Geometry check sheet. Reference: drawing and pictorial views, mm from the part's lowest x, y, z. A direction names the side the tool comes from. Round coordinates to 2 decimals unless told otherwise and drop trailing zeros. Write each loop counter-clockwise with the first axis right and the second up, starting at its lowest first coordinate (ties: lowest second). Pieces come first, ordered by that corner, then holes. Notation, with made-up numbers: M 57,-31 L 85,-31 A12 ccw 85,-23 Z; hole C -23.75,-36 d7. An arc over 180 degrees is marked long. Answer in a Markdown table with one row per item.
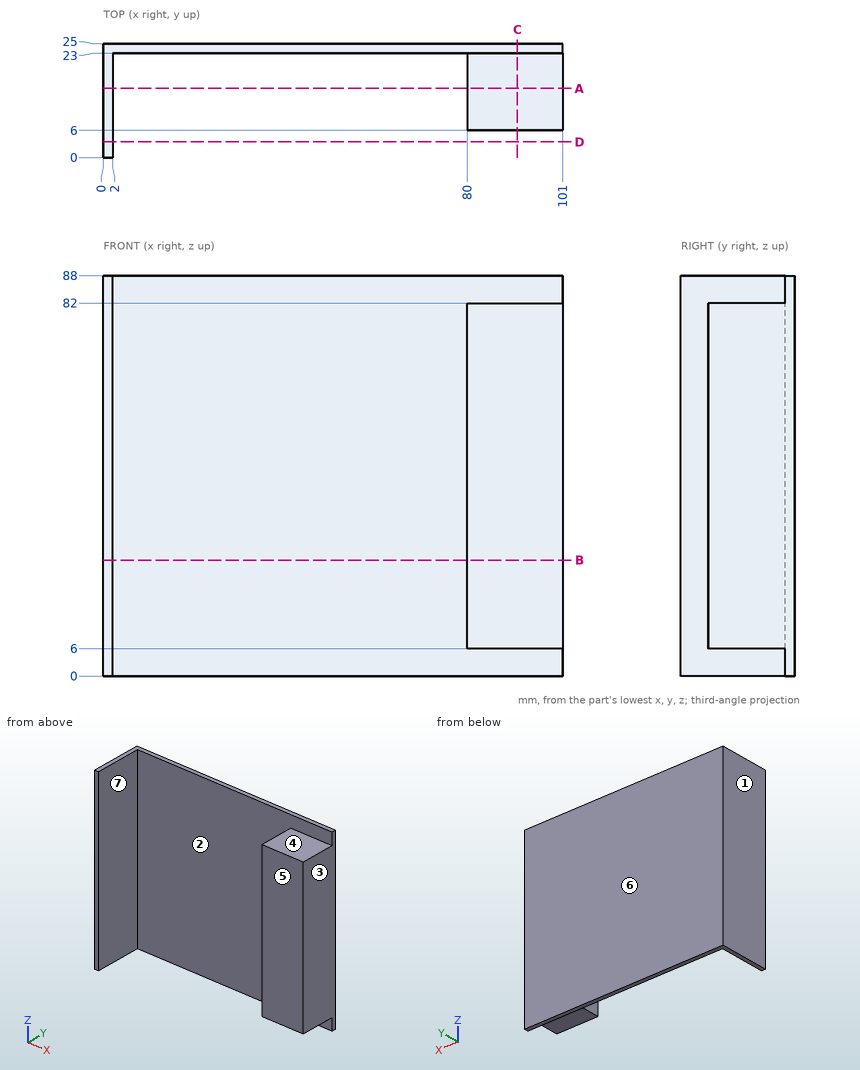
1. Section check C-C, the plane x = 91. Record the cut outline in (y, z).
Found:
| item | result |
|---|---|
| outline | M 6,6 L 23,6 L 23,0 L 25,0 L 25,88 L 23,88 L 23,82 L 6,82 Z |
2. Draft check along X on the marked faces 1, 2, 3 and 4. Enter one of: +X half, -X half, draft (parallel to the pull), parting line (faces both ways), or undercut.
Found:
| item | result |
|---|---|
| face 1 | -X half |
| face 2 | undercut |
| face 3 | +X half |
| face 4 | draft |
3. Section check A-A, the plane y = 15.25. Record the cut outline in (x, z), and give its area (3 significant figures).
Found:
| item | result |
|---|---|
| outline | M 0,0 L 2,0 L 2,88 L 0,88 Z; M 80,6 L 101,6 L 101,82 L 80,82 Z |
| area | 1,770 mm2 |
4. Access from +Z, -Z, +X, -X, +Y, -Y to the whole of each face (thin tool, end or side, straight path). Record for the marked faces 5, 6 and 7.
Found:
| item | result |
|---|---|
| face 5 | +Z, -Z, +X, -Y |
| face 6 | +Z, -Z, +X, -X, +Y |
| face 7 | +Z, -Z, -Y |
5. Section check B-B, the plane z = 25.5. Record the cut outline in (x, y).
Found:
| item | result |
|---|---|
| outline | M 0,0 L 2,0 L 2,23 L 80,23 L 80,6 L 101,6 L 101,25 L 0,25 Z |
6. Go/stop test with flat-tipped pins: pin 1 (13.5 mm diameter, centred on x = 85.5, y = 13.5, fed in from +Z); pin 2 (13.5 mm diameter, centred on x = 94, y = 14, fed in from -Z); pin 3 (8 mm diameter, centred on x = 65.5, z = 29.5, fed in from -Y). Record where each tip stops, or that it passes through.
Found:
| item | result |
|---|---|
| pin 1 | stops at z = 82 |
| pin 2 | stops at z = 6 |
| pin 3 | stops at y = 23 |
7. Scan lines: L1, parallel to X at y = 12.25, z = 45.5; L2, parallel to Z at x = 89.5, y = 7.25; L3, parallel to X at y = 4.75, z = 34. Record each from-to range of solid material in increasing order.
Found:
| item | result |
|---|---|
| L1 | x = 0 to 2, 80 to 101 |
| L2 | z = 6 to 82 |
| L3 | x = 0 to 2 |
8. Section check D-D, the plane y = 3.5. Record the cut outline in (x, z).
Found:
| item | result |
|---|---|
| outline | M 0,0 L 2,0 L 2,88 L 0,88 Z |
